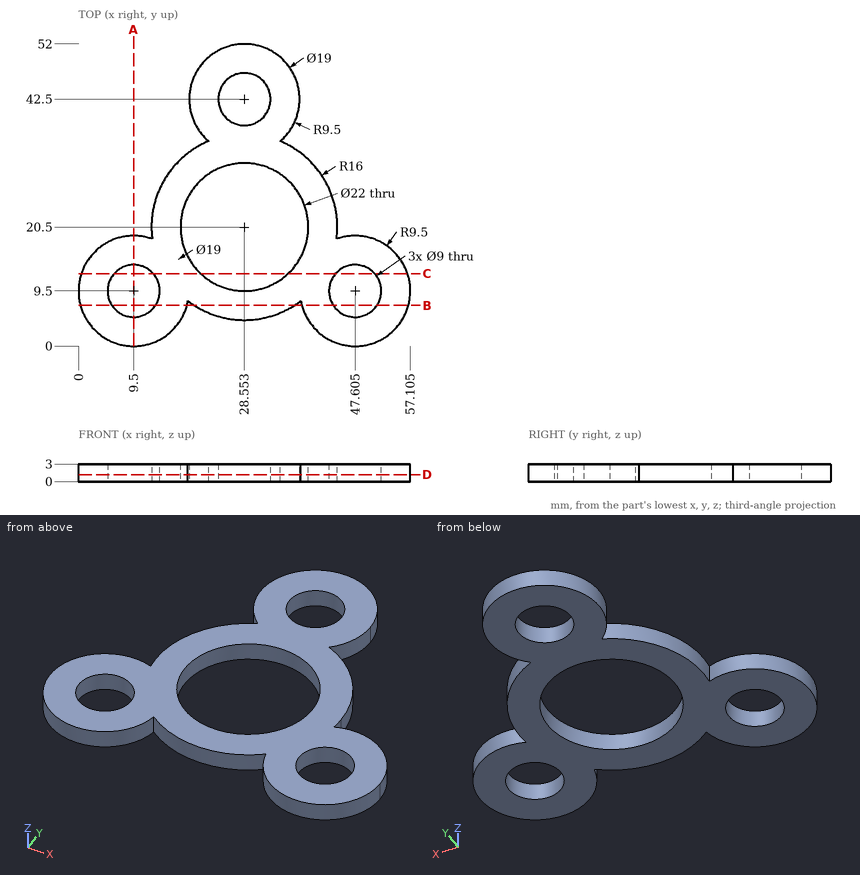
Source: three-view drawing plus pictorial views. Frame: mm from the lowest corner of the part. Give positions to 0.01 mm unless a question says otherwise; leave off trailing zeros. Loops run counter-clockwise (first coordinate to the right, second up) from the corner with the lowest first, then second, coordinate; pieces in that order, holes last. Notation, with made-up numbers: (-20, -28) -> (-13, -28) arc R21 ccw to (-13, -24) -> close; hole circle Ø9 at (-16.75, 89). An arc over 180 degrees is marked (long way). Use a Markdown table: item, result. Add a question column.
(1) Ray query, line 1 (Y direction, x = 21, z = 1.45) (1 decimal); line 2 (Y direction, x = 30, z = 2.15) (1 decimal); line 3 (Y direction, x = 9.5, z = 1.9). Return the intervals inside material, ascending.
(2) Section query D-D (z = 1.2). Count the separate pieces of the cut face and the enclosed holes in it, then the cut area to 3 significant figures.
(3) Section query C-C (y = 12.5). Output: boundary loops of the cut face in (x, z).
(4) First-contact query: pin 1 Ø5.5 at (x, y) = (9.5, 9.5) entering from -Z. Flat tip, straight axial feed; report the tip coordinate or a pass-through.
(5) Section query A-A (x = 9.5). Output: boundary loops of the cut face in (y, z).
(6) Section query B-B (y = 7). Output: boundary loops of the cut face in (x, z) (1 decimal).
Checked values:
| question | item | result |
|---|---|---|
| 1 | line 1 | 6.4 to 12.5, 28.5 to 34.6, 36.7 to 48.3 |
| 1 | line 2 | 4.6 to 9.6, 31.4 to 38.2, 46.8 to 51.9 |
| 1 | line 3 | 0 to 5, 14 to 19 |
| 2 | separate pieces | 1 |
| 2 | enclosed holes | 4 |
| 2 | area | 996 mm^2 |
| 3 | outline | (0.49, 0) -> (6.15, 0) -> (6.15, 3) -> (0.49, 3) -> close; (12.85, 0) -> (21, 0) -> (21, 3) -> (12.85, 3) -> close; (36.1, 0) -> (44.25, 0) -> (44.25, 3) -> (36.1, 3) -> close; (50.96, 0) -> (56.62, 0) -> (56.62, 3) -> (50.96, 3) -> close |
| 4 | pin 1 | through |
| 5 | outline | (0, 0) -> (5, 0) -> (5, 3) -> (0, 3) -> close; (14, 0) -> (19, 0) -> (19, 3) -> (14, 3) -> close |
| 6 | outline | (0.3, 0) -> (5.8, 0) -> (5.8, 3) -> (0.3, 3) -> close; (13.2, 0) -> (18.7, 0) -> (18.7, 3) -> (13.2, 3) -> close; (20, 0) -> (37.1, 0) -> (37.1, 3) -> (20, 3) -> close; (38.4, 0) -> (43.9, 0) -> (43.9, 3) -> (38.4, 3) -> close; (51.3, 0) -> (56.8, 0) -> (56.8, 3) -> (51.3, 3) -> close |
